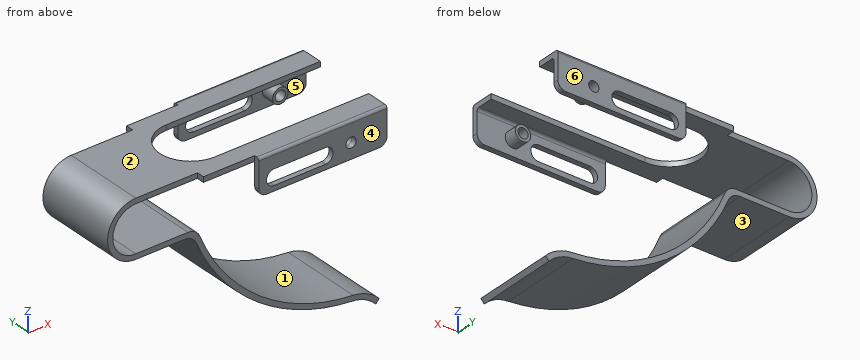
```python
from build123d import *

# Parameters (mm, degrees)
F1_DEPTH  = 16
F2_W      = 70
F2_H      = 3
F3_DEPTH  = 2
F4_W      = 50
F4_H      = 14
F5_DEPTH  = 2
F6_R      = 1
F9_DEPTH  = 2
F11_DEPTH = 42.001
F13_D     = 4
F14_R     = 3
F14_R_2   = 2
F15_DEPTH = 5
F16_R     = 3


# Not quite as in the source:
# - a pattern or mirror of a feature is missing from the dataset's text; its kind, count and spacing are read off the source's solid


with BuildPart() as f1:
    # F0 (on Front) → F1 (new body)
    with BuildSketch(Plane.XZ):
        with BuildLine():
            ThreePointArc((0, -9), (-9, 0), (0, 9))
            Line((0, 9), (94, 9))
            Line((94, 9), (94, 11))
            Line((94, 11), (0, 11))
            ThreePointArc((0, 11), (-11, 0), (0, -11))
            Line((0, -11), (19, -11))
            ThreePointArc((19, -11), (21.7681124643, -11.8361612201), (23.6103896104, -14.064978646))
            ThreePointArc((23.6103896104, -14.064978646), (47.704208574, -44.4678662727), (84.0759449666, -57.9565459739))
            ThreePointArc((84.0759449666, -57.9565459739), (89.2804195373, -59.3196982134), (93.5865207758, -62.5449473062))
            Line((93.5865207758, -62.5449473062), (94.8828854905, -61))
            ThreePointArc((94.8828854905, -61), (90.2510294077, -57.5678191663), (84.7034264019, -56))
            ThreePointArc((84.7034264019, -56), (48.5673164119, -42.6217020739), (24.9861322889, -12.1467114099))
            ThreePointArc((24.9861322889, -12.1467114099), (23.1470623984, -9.8607704249), (20.3422845953, -9))
            Line((20.3422845953, -9), (0, -9))
        make_face()
    extrude(amount=F1_DEPTH)

    # F2 (on face) → F3 (join)
    with BuildSketch(Plane.XY.offset(11)):
        with Locations((59, -17.5)):
            Rectangle(F2_W, F2_H)
    extrude(amount=-F3_DEPTH)

    # F4 (on face) → F5 (join)
    with BuildSketch(Plane.XZ.offset(19)):
        with Locations((69, 4)):
            Rectangle(F4_W, F4_H)
    extrude(amount=F5_DEPTH)

    # F6
    f6_edges = [f1.edges().sort_by_distance(p)[0] for p in [
        (69, -21, 11),
        (69, -19, 9),
    ]]
    fillet(f6_edges, radius=F6_R)

    # F7: F1 across plane


with BuildPart() as f1_1:
    add(f1.part)
    add(f1.part.mirror(Plane.XZ))

    # F8 (on face) → F9 (cut)
    with BuildSketch(Plane.XY.offset(11)):
        with BuildLine():
            Line((94, 12), (34, 12))
            ThreePointArc((34, 12), (22, 0), (34, -12))
            Line((34, -12), (94, -12))
            Line((94, -12), (94, 12))
        make_face()
    extrude(amount=-F9_DEPTH, mode=Mode.SUBTRACT)

    # F10 (on face) → F11 (cut, through all)
    with BuildSketch(Plane.XZ.offset(21)):
        with BuildLine():
            ThreePointArc((50, 5), (47, 2), (50, -1))
            Line((50, -1), (70, -1))
            ThreePointArc((70, -1), (73, 2), (70, 5))
            Line((70, 5), (50, 5))
        make_face()
    extrude(amount=-F11_DEPTH, mode=Mode.SUBTRACT)

    # F13 (through all)
    with Locations(Plane.XZ.offset(21)):
        with Locations((80, 3)):
            Hole(F13_D / 2)

    # F14 (on face) → F15 (join)
    with BuildSketch(Plane(origin=(0, -19, 0), x_dir=(-1, 0, 0), z_dir=(0, 1, 0))):
        with Locations((-80, 3)):
            Circle(F14_R)
        with Locations((-80, 3)):
            Circle(F14_R_2, mode=Mode.SUBTRACT)
    f15 = extrude(amount=F15_DEPTH)

    # F15_copies: F15 across plane
    add(f15.mirror(Plane.ZX))

    # F16
    f16_edges = [f1_1.edges().sort_by_distance(p)[0] for p in [
        (94, 20, -3),
        (44, 20, -3),
        (44, -20, -3),
        (94, -20, -3),
    ]]
    fillet(f16_edges, radius=F16_R)


solid = f1_1.part
```
The model under review builds one solid part; all positions refer to its coordinate system, in mm. Face numbers are marked on the shaded views. A direction names the side the tool comes from. Give positions to 0.01 mm unless a question says otherwise; leave off trailing zeros. Write each loop counter-clockwise with the first axis right and the second up, starting at its lowest first coordinate (ties: lowest second). Pieces come first, ordered by that corner, then holes. Notation, with made-up numbers: M 88,16.25 L 94,16.25 A14 cw 94,31.25 Z; hole C 3.5,86.5 d3. An arc over 180 degrees is marked long. Answer in a Markdown table with one row per item.
Item 1: Tool access review of the marked faces 1, 2 and 3: name each direction out of +Z, -Z, +X, -X, +Y, -Y from which nothing blocks a thin tool from reaching the whole face with its end or side.
Check sheet entries:
| item | result |
|---|---|
| face 1 | +X, +Y, -Y |
| face 2 | +Z, +X, -X, +Y, -Y |
| face 3 | -Z, -X, +Y, -Y |
Item 2: For P1, Ø3, axis at y = -11, z = -19, coming from the -X side; P2, Ø2, axis at x = 34.5, z = 9.5, coming from the -Y side; P3, Ø0.9, axis at y = -20, z = 3.5, coming from the -X side, all flat-tipped, find the tip position at first contact; note any pin that passes through.
Check sheet entries:
| item | result |
|---|---|
| P1 | x = 25.16 |
| P2 | y = -19 |
| P3 | x = 44 |
Item 3: Add section C-C on x = 15. Give the boundary of the cut face in (y, z).
Check sheet entries:
| item | result |
|---|---|
| outline | M -16,-11 L 16,-11 L 16,-9 L -16,-9 Z; M -16,9 L 16,9 L 16,11 L -16,11 Z |
Item 4: For line 1 along Y through (x, z) = (87.5, 2); line 2 along Z through (x, y) = (14.5, -11); line 3 along Z through (x, y) = (41, 18), list the stretches that pass through material, from the lowest coordinate up.
Check sheet entries:
| item | result |
|---|---|
| line 1 | -21 to -19, 19 to 21 |
| line 2 | -11 to -9, 9 to 11 |
| line 3 | 9 to 11 |
Item 5: Add section B-B on y = 0. Give the boundary of the cut face in (x, z).
Check sheet entries:
| item | result |
|---|---|
| outline | M 0,-11 L 19,-11 A5 cw 23.61,-14.06 A72 ccw 84.08,-57.96 A14 cw 93.59,-62.54 L 94.88,-61 A16 ccw 84.7,-56 A70 cw 24.99,-12.15 A5 ccw 20.34,-9 L 0,-9 A9 cw 0,9 L 22,9 L 22,11 L 0,11 A11 ccw Z |
Item 6: Add section A-A on x = 56.5. Give the boundary of the cut face in (y, z).
Check sheet entries:
| item | result |
|---|---|
| outline | M -21,-3 L -19,-3 L -19,-1 L -21,-1 Z; M -21,5 L -19,5 L -19,8 A1 cw -18,9 L -12,9 L -12,11 L -20,11 A1 ccw -21,10 Z; M -16,-49.93 L 16,-49.93 L 16,-47.66 L -16,-47.66 Z; M 12,9 L 18,9 A1 cw 19,8 L 19,5 L 21,5 L 21,10 A1 ccw 20,11 L 12,11 Z; M 19,-3 L 21,-3 L 21,-1 L 19,-1 Z |
Item 7: Add section D-D on x = 45.5. Give the boundary of the cut face in (y, z), plus the area to 3 significant figures.
Check sheet entries:
| item | result |
|---|---|
| outline | M -21,-2.6 L -19,-2.6 L -19,8 A1 cw -18,9 L -12,9 L -12,11 L -20,11 A1 ccw -21,10 Z; M -16,-42.8 L 16,-42.8 L 16,-40.24 L -16,-40.24 Z; M 12,9 L 18,9 A1 cw 19,8 L 19,-2.6 L 21,-2.6 L 21,10 A1 ccw 20,11 L 12,11 Z |
| area | 165 mm2 |
Item 8: Draft analysis for pull direction Y (two halves, no side actions). For the marked faces 4, 5 and 6, state which applies: +Y half, -Y half, draft (parallel to the pull), parting line (faces both ways), or undercut.
Check sheet entries:
| item | result |
|---|---|
| face 4 | -Y half |
| face 5 | undercut |
| face 6 | +Y half |
